```python
from build123d import *

# Parameters (mm, degrees)
F0_W     = 250
F0_H     = 200
F1_DEPTH = 300
F2_W     = 230
F2_H     = 20
F3_DEPTH = 280
F4_W     = 230
F4_H     = 55
F5_DEPTH = 30
F6_R     = 37.5
F7_DEPTH = 160
F6_W     = 40
F6_H     = 75
F8_DEPTH = 200


with BuildPart() as f1:
    # F0 (on Top) → F1 (new body)
    with BuildSketch(Plane.XY):
        with Locations((0.84289, 5.342618)):
            Rectangle(F0_W, F0_H)
    extrude(amount=F1_DEPTH)

    # F2 (on face) → F3 (cut)
    with BuildSketch(Plane.XY.offset(300)):
        with Locations((0.84289, 85.342618)):
            Rectangle(F2_W, F2_H)
        with Locations((0.84289, 60.342618)):
            Rectangle(F2_W, F2_H)
        with Locations((0.84289, 35.342618)):
            Rectangle(F2_W, F2_H)
        with Locations((0.84289, 10.342618)):
            Rectangle(F2_W, F2_H)
    extrude(amount=-F3_DEPTH, mode=Mode.SUBTRACT)

    # F4 (on face) → F5 (cut)
    with BuildSketch(Plane.XY.offset(300)):
        with Locations((0.84289, 47.842618)):
            Rectangle(F4_W, F4_H)
    extrude(amount=-F5_DEPTH, mode=Mode.SUBTRACT)

    # F6 (on face) → F7 (cut)
    with BuildSketch(Plane.XY.offset(300)):
        with Locations((77.84289, -47.157382)):
            Circle(F6_R)
    extrude(amount=-F7_DEPTH, mode=Mode.SUBTRACT)

    # F6 (on face) → F8 (cut)
    with BuildSketch(Plane.XY.offset(300)):
        with Locations((-94.15711, -47.157382)):
            Rectangle(F6_W, F6_H)
        Polygon((-19.15711, -84.657382), (-69.15711, -9.657382), (-69.15711, -84.657382), align=None)
        Polygon((-13.147858, -9.657382), (-63.147858, -9.657382), (-13.147858, -84.657382), align=None)
        Polygon((-8.147858, -9.657382), (-8.147858, -84.657382), (41.852142, -84.657382), align=None)
        with BuildLine():
            Line((36.611834, -9.657382), (-2.138606, -9.657382))
            Line((-2.138606, -9.657382), (21.415755, -44.988925))
            ThreePointArc((21.415755, -44.988925), (26.797834, -47.06384), (30.553805, -42.686086))
            ThreePointArc((30.553805, -42.686086), (33.747208, -29.498932), (40.538601, -17.752621))
            ThreePointArc((40.538601, -17.752621), (41.110511, -12.475204), (36.611834, -9.657382))
        make_face()
    extrude(amount=-F8_DEPTH, mode=Mode.SUBTRACT)


solid = f1.part
```
Source: CAD feature listing. Evaluate the final solid. Frame: model axes, mm. A direction names the side the tool comes from. Coordinates: 2 decimals unless noted, no trailing zeros. Loops run counter-clockwise (first coordinate to the right, second up) from the corner with the lowest first, then second, coordinate; pieces in that order, holes last. Notation, with made-up numbers: (55.5, 77.5) -> (96.5, 77.5) arc R22 ccw to (96.5, 107.5) -> close; hole circle Ø2 at (68, 8). An arc over 180 degrees is marked (long way). One line per item, written item: value. Start each with the question number.
Q1. Line query: line 1 along Y through (x, z) = (82, 38); line 2 along Y through (x, z) = (-108.5, 130); line 3 along Y through (x, z) = (79, 205). Output: solid intervals per line, ascending.
Q2. Section query A-A, the plane y = 85. Return the cut outline in (x, z), and give its area (3 significant figures).
Q3. Section query D-D, the plane x = 93. Return the cut outline in (y, z), and give its area (3 significant figures).
Q4. Contact query for flat-ended pins moving along their axis: P1, Ø6, axis at x = 40.5, y = 12.5, coming from the +Z side; P2, Ø3, axis at x = 27, y = 46, coming from the +Z side. Output: stop coordinate, or through.
Q5. Set-up query: faces 1 (the face through (-1, 7, 0)), 2 (the face through (-69.157, -47, 201)). Return all of +Z, -Z, +X, -X, +Y, -Y with unobstructed straight access to the full face (end or side cutting, diameter ignored); none if empty.
Q6. Mould query, pull axis Y, two halves, no side actions, for faces 3 (the face through (125.843, 4, 148)), 4 (the face through (18, -9.657, 201)). Classes: pulls with the +Y half, pulls with the -Y half, needs draft (parallel to the pull), parting line crosses it, or undercut.
Q7. Section query B-B, the plane x = 4. Return the cut outline in (y, z), and give its area (3 significant figures).
Q8. Section query C-C, the plane z = 204. Give the number of separate pieces and of enclosed holes in the cut face, and give its area (3 significant figures).
Results:
1. line 1: -94.66 to 0.34, 20.34 to 25.34, 45.34 to 50.34, 70.34 to 75.34, 95.34 to 105.34
1. line 2: -94.66 to -84.66, -9.66 to 0.34, 20.34 to 25.34, 45.34 to 50.34, 70.34 to 75.34, 95.34 to 105.34
1. line 3: -94.66 to -84.64, -9.68 to 0.34, 20.34 to 25.34, 45.34 to 50.34, 70.34 to 75.34, 95.34 to 105.34
2. outline: (-124.16, 0) -> (125.84, 0) -> (125.84, 300) -> (115.84, 300) -> (115.84, 20) -> (-114.16, 20) -> (-114.16, 300) -> (-124.16, 300) -> close
2. area: 10,600 mm^2
3. outline: (-94.66, 0) -> (105.34, 0) -> (105.34, 300) -> (95.34, 300) -> (95.34, 20) -> (75.34, 20) -> (75.34, 270) -> (70.34, 270) -> (70.34, 20) -> (50.34, 20) -> (50.34, 270) -> (45.34, 270) -> (45.34, 20) -> (25.34, 20) -> (25.34, 270) -> (20.34, 270) -> (20.34, 20) -> (0.34, 20) -> (0.34, 300) -> (-12.86, 300) -> (-12.86, 140) -> (-81.46, 140) -> (-81.46, 300) -> (-94.66, 300) -> close
3. area: 26,200 mm^2
4. P1: z = 20
4. P2: z = 270
5. face 1: -Z, +X, -X, +Y, -Y
5. face 2: +Z
6. face 3: needs draft
6. face 4: undercut
7. outline: (-94.66, 0) -> (105.34, 0) -> (105.34, 300) -> (95.34, 300) -> (95.34, 20) -> (75.34, 20) -> (75.34, 270) -> (70.34, 270) -> (70.34, 20) -> (50.34, 20) -> (50.34, 270) -> (45.34, 270) -> (45.34, 20) -> (25.34, 20) -> (25.34, 270) -> (20.34, 270) -> (20.34, 20) -> (0.34, 20) -> (0.34, 300) -> (-9.66, 300) -> (-9.66, 100) -> (-18.87, 100) -> (-18.87, 300) -> (-27.88, 300) -> (-27.88, 100) -> (-84.66, 100) -> (-84.66, 300) -> (-94.66, 300) -> close
7. area: 24,000 mm^2
8. separate pieces: 1
8. enclosed holes: 10
8. area: 17,600 mm^2
